from build123d import *

# Parameters (mm, degrees)
F0_R     = 2.1
F1_DEPTH = 1500


with BuildPart() as f1:
    # F0 (on Top) → F1 (new body)
    with BuildSketch(Plane.XY):
        with BuildLine():
            Line((-3.4, 0), (-3.5, -0.1))
            Line((-3.5, -0.1), (-3.5, -2.43934))
            Line((-3.5, -2.43934), (-6.56066, -5.5))
            Line((-6.56066, -5.5), (-8.2, -5.5))
            Line((-8.2, -5.5), (-8.2, -2.89))
            Line((-8.2, -2.89), (-8.31, -2.89))
            Line((-8.31, -2.89), (-9.768614, -4.348614))
            ThreePointArc((-9.768614, -4.348614), (-9.939865, -4.604909), (-10, -4.907229))
            Line((-10, -4.907229), (-10, -8.5))
            ThreePointArc((-10, -8.5), (-9.56066, -9.56066), (-8.5, -10))
            Line((-8.5, -10), (-4.907229, -10))
            ThreePointArc((-4.907229, -10), (-4.604909, -9.939865), (-4.348614, -9.768614))
            Line((-4.348614, -9.768614), (-2.89, -8.31))
            Line((-2.89, -8.31), (-2.89, -8.2))
            Line((-2.89, -8.2), (-5.5, -8.2))
            Line((-5.5, -8.2), (-5.5, -6.56066))
            Line((-5.5, -6.56066), (-2.43934, -3.5))
            Line((-2.43934, -3.5), (-0.1, -3.5))
            Line((-0.1, -3.5), (0, -3.4))
            Line((0, -3.4), (0.1, -3.5))
            Line((0.1, -3.5), (2.43934, -3.5))
            Line((2.43934, -3.5), (5.5, -6.56066))
            Line((5.5, -6.56066), (5.5, -8.2))
            Line((5.5, -8.2), (2.89, -8.2))
            Line((2.89, -8.2), (2.89, -8.31))
            Line((2.89, -8.31), (4.348614, -9.768614))
            ThreePointArc((4.348614, -9.768614), (4.604909, -9.939865), (4.907229, -10))
            Line((4.907229, -10), (10, -10))
            Line((10, -10), (15.092771, -10))
            ThreePointArc((15.092771, -10), (15.395091, -9.939865), (15.651386, -9.768614))
            Line((15.651386, -9.768614), (17.11, -8.31))
            Line((17.11, -8.31), (17.11, -8.2))
            Line((17.11, -8.2), (14.5, -8.2))
            Line((14.5, -8.2), (14.5, -6.56066))
            Line((14.5, -6.56066), (17.56066, -3.5))
            Line((17.56066, -3.5), (19.9, -3.5))
            Line((19.9, -3.5), (20, -3.4))
            Line((20, -3.4), (20.1, -3.5))
            Line((20.1, -3.5), (22.43934, -3.5))
            Line((22.43934, -3.5), (25.5, -6.56066))
            Line((25.5, -6.56066), (25.5, -8.2))
            Line((25.5, -8.2), (22.89, -8.2))
            Line((22.89, -8.2), (22.89, -8.31))
            Line((22.89, -8.31), (24.348614, -9.768614))
            ThreePointArc((24.348614, -9.768614), (24.604909, -9.939865), (24.907229, -10))
            Line((24.907229, -10), (28.5, -10))
            ThreePointArc((28.5, -10), (29.56066, -9.56066), (30, -8.5))
            Line((30, -8.5), (30, -4.907229))
            ThreePointArc((30, -4.907229), (29.939865, -4.604909), (29.768614, -4.348614))
            Line((29.768614, -4.348614), (28.31, -2.89))
            Line((28.31, -2.89), (28.2, -2.89))
            Line((28.2, -2.89), (28.2, -5.5))
            Line((28.2, -5.5), (26.56066, -5.5))
            Line((26.56066, -5.5), (23.5, -2.43934))
            Line((23.5, -2.43934), (23.5, -0.1))
            Line((23.5, -0.1), (23.4, 0))
            Line((23.4, 0), (23.5, 0.1))
            Line((23.5, 0.1), (23.5, 2.43934))
            Line((23.5, 2.43934), (26.56066, 5.5))
            Line((26.56066, 5.5), (28.2, 5.5))
            Line((28.2, 5.5), (28.2, 2.89))
            Line((28.2, 2.89), (28.31, 2.89))
            Line((28.31, 2.89), (29.768614, 4.348614))
            ThreePointArc((29.768614, 4.348614), (29.939865, 4.604909), (30, 4.907229))
            Line((30, 4.907229), (30, 8.5))
            ThreePointArc((30, 8.5), (29.56066, 9.56066), (28.5, 10))
            Line((28.5, 10), (24.907229, 10))
            ThreePointArc((24.907229, 10), (24.604909, 9.939865), (24.348614, 9.768614))
            Line((24.348614, 9.768614), (22.89, 8.31))
            Line((22.89, 8.31), (22.89, 8.2))
            Line((22.89, 8.2), (25.5, 8.2))
            Line((25.5, 8.2), (25.5, 6.56066))
            Line((25.5, 6.56066), (22.43934, 3.5))
            Line((22.43934, 3.5), (20.1, 3.5))
            Line((20.1, 3.5), (20, 3.4))
            Line((20, 3.4), (19.9, 3.5))
            Line((19.9, 3.5), (17.56066, 3.5))
            Line((17.56066, 3.5), (14.5, 6.56066))
            Line((14.5, 6.56066), (14.5, 8.2))
            Line((14.5, 8.2), (17.11, 8.2))
            Line((17.11, 8.2), (17.11, 8.31))
            Line((17.11, 8.31), (15.651386, 9.768614))
            ThreePointArc((15.651386, 9.768614), (15.395091, 9.939865), (15.092771, 10))
            Line((15.092771, 10), (10, 10))
            Line((10, 10), (4.907229, 10))
            ThreePointArc((4.907229, 10), (4.604909, 9.939865), (4.348614, 9.768614))
            Line((4.348614, 9.768614), (2.89, 8.31))
            Line((2.89, 8.31), (2.89, 8.2))
            Line((2.89, 8.2), (5.5, 8.2))
            Line((5.5, 8.2), (5.5, 6.56066))
            Line((5.5, 6.56066), (2.43934, 3.5))
            Line((2.43934, 3.5), (0.1, 3.5))
            Line((0.1, 3.5), (0, 3.4))
            Line((0, 3.4), (-0.1, 3.5))
            Line((-0.1, 3.5), (-2.43934, 3.5))
            Line((-2.43934, 3.5), (-5.5, 6.56066))
            Line((-5.5, 6.56066), (-5.5, 8.2))
            Line((-5.5, 8.2), (-2.89, 8.2))
            Line((-2.89, 8.2), (-2.89, 8.31))
            Line((-2.89, 8.31), (-4.348614, 9.768614))
            ThreePointArc((-4.348614, 9.768614), (-4.604909, 9.939865), (-4.907229, 10))
            Line((-4.907229, 10), (-8.5, 10))
            ThreePointArc((-8.5, 10), (-9.56066, 9.56066), (-10, 8.5))
            Line((-10, 8.5), (-10, 4.907229))
            ThreePointArc((-10, 4.907229), (-9.939865, 4.604909), (-9.768614, 4.348614))
            Line((-9.768614, 4.348614), (-8.31, 2.89))
            Line((-8.31, 2.89), (-8.2, 2.89))
            Line((-8.2, 2.89), (-8.2, 5.5))
            Line((-8.2, 5.5), (-6.56066, 5.5))
            Line((-6.56066, 5.5), (-3.5, 2.43934))
            Line((-3.5, 2.43934), (-3.5, 0.1))
            Line((-3.5, 0.1), (-3.4, 0))
        make_face()
        Polygon((-7.66, -6.57), (-7.115, -7.115), (-6.57, -7.66), (-6.57, -8.2), (-8.2, -8.2), (-8.2, -6.57), align=None, mode=Mode.SUBTRACT)
        Polygon((27.115, -7.115), (27.66, -6.57), (28.2, -6.57), (28.2, -8.2), (26.57, -8.2), (26.57, -7.66), align=None, mode=Mode.SUBTRACT)
        Circle(F0_R, mode=Mode.SUBTRACT)
        Polygon((-6.57, 8.2), (-6.57, 7.66), (-7.115, 7.115), (-7.66, 6.57), (-8.2, 6.57), (-8.2, 8.2), align=None, mode=Mode.SUBTRACT)
        Polygon((3.5, -2.43934), (3.5, -0.1), (3.4, 0), (3.5, 0.1), (3.5, 2.43934), (6.9, 5.83934), (6.9, 8.2), (10, 8.2), (13.1, 8.2), (13.1, 5.83934), (16.5, 2.43934), (16.5, 0.1), (16.6, 0), (16.5, -0.1), (16.5, -2.43934), (13.1, -5.83934), (13.1, -8.2), (10, -8.2), (6.9, -8.2), (6.9, -5.83934), align=None, mode=Mode.SUBTRACT)
        with Locations((20, 0)):
            Circle(F0_R, mode=Mode.SUBTRACT)
        Polygon((27.66, 6.57), (27.115, 7.115), (26.57, 7.66), (26.57, 8.2), (28.2, 8.2), (28.2, 6.57), align=None, mode=Mode.SUBTRACT)
    extrude(amount=F1_DEPTH)


solid = f1.part
Read the model definition and answer for the solid it produces. Units are mm, in the model's axes. Coordinates: 2 decimals unless noted, no trailing zeros. Answer as a JSON object with one key per item and string values.
1) A cutting plane is placed at A-A, the plane z = 644. State how many separate pieces and enclosed holes the cut face has, plus the area to 3 significant figures.
Model answer:
{"separate pieces": "1", "enclosed holes": "7", "area": "270 mm²"}
2) Each of these flat-tipped pins is pushed along its axis until it touches: pin 1 (1 mm diameter, centred on x = -4, z = 1204.5, fed in from -Y); pin 2 (0.8 mm diameter, centred on x = 16, z = 523, fed in from +Y); pin 3 (3 mm diameter, centred on x = 25.5, y = 0.5, fed in from +Z); pin 4 (5 mm diameter, centred on x = 21, z = 1243.5, fed in from -Y). Where does it stop, or does it pass through?
Model answer:
{"pin 1": "stops at y = -9.89", "pin 2": "stops at y = 9.82", "pin 3": "passes through", "pin 4": "stops at y = -8.92"}
3) Consider line 1 along X through (y, z) = (-6.25, 1307); line 2 along X through (y, z) = (4.5, 505); line 3 along Y through (x, z) = (15.5, 689.5). Determine where each line is inside the solid, lowest interval first. Write a range as from..to.
Model answer:
{"line 1": "x = -10..-5.19, 5.19..6.9, 13.1..14.81, 25.19..30", "line 2": "x = -9.89..-8.2, -5.56..-3.44, 3.44..5.56, 14.44..16.56, 23.44..25.56, 28.2..29.89", "line 3": "y = -9.89..-8.2, -5.56..-3.44, 3.44..5.56, 8.2..9.89"}
